Check sheet for the modelled part. Datum: model origin and axes. Units: mm. Coordinates: 2 decimals unless noted, no trailing zeros. Loops run counter-clockwise (first coordinate to the right, second up) from the corner with the lowest first, then second, coordinate; pieces in that order, holes last. Notation, with made-up numbers: (-1.75, -38.5) -> (22.25, -38.5) arc R10 ccw to (22.25, -26.5) -> close; hole circle Ø11 at (36.25, 12.25). An arc over 180 degrees is marked (long way). Use CSV: the item, a comma, the result in double quotes.
```python
from build123d import *

# Parameters (mm, degrees)
SKIZZE1_R                            = 20.35
SKIZZE1_R_2                          = 19
AUFSATZ_LINEAR_AUSTRAGEN1_DEPTH      = 170
SKIZZE2_R                            = 2.5
SCHNITT_LINEAR_AUSTRAGEN1_DEPTH      = 21.35
SCHNITT_LINEAR_AUSTRAGEN1_DEPTH_BACK = 21.35
SKIZZE3_R                            = 2.5
SCHNITT_LINEAR_AUSTRAGEN2_DEPTH      = 21.3500001
SCHNITT_LINEAR_AUSTRAGEN2_DEPTH_BACK = 21.3500001


with BuildPart() as part:
    # Skizze1 → Aufsatz-Linear austragen1 (new body)
    with BuildSketch(Plane(origin=(0, 0, 0), x_dir=(1, 0, 0), z_dir=(0, 1, 0))):
        Circle(SKIZZE1_R)
        Circle(SKIZZE1_R_2, mode=Mode.SUBTRACT)
    extrude(amount=AUFSATZ_LINEAR_AUSTRAGEN1_DEPTH)

    # Skizze2 → Schnitt-Linear austragen1 (cut, two sides)
    with BuildSketch(Plane.XY) as schnitt_linear_austragen1_sk:
        with Locations((0, 162.5)):
            Circle(SKIZZE2_R)
    extrude(amount=SCHNITT_LINEAR_AUSTRAGEN1_DEPTH, mode=Mode.SUBTRACT)
    extrude(schnitt_linear_austragen1_sk.sketch, amount=-SCHNITT_LINEAR_AUSTRAGEN1_DEPTH_BACK, mode=Mode.SUBTRACT)

    # Skizze3 → Schnitt-Linear austragen2 (cut, two sides)
    with BuildSketch(Plane(origin=(0, 0, 0), x_dir=(0, 0, -1), z_dir=(1, 0, 0))) as schnitt_linear_austragen2_sk:
        with Locations((0, 162.5)):
            Circle(SKIZZE3_R)
    extrude(amount=SCHNITT_LINEAR_AUSTRAGEN2_DEPTH, mode=Mode.SUBTRACT)
    extrude(schnitt_linear_austragen2_sk.sketch, amount=-SCHNITT_LINEAR_AUSTRAGEN2_DEPTH_BACK, mode=Mode.SUBTRACT)


solid = part.part
```
1) Cross-section at C-C on z = -9. Record the boundary of the cut face in (x, y).
Answer below:
outline,"(-18.25, 0) -> (-16.73, 0) -> (-16.73, 170) -> (-18.25, 170) -> close; (16.73, 0) -> (18.25, 0) -> (18.25, 170) -> (16.73, 170) -> close"
2) Draft check along Y on faces 1 (the flat face through (-17, 170, -9)), 2 (the flat face through (-17, 0, -9)), 3 (the cylindrical face through (20, 165, 0)). Enter one of: released by +Y, released by -Y, zero draft, split by the parting line, or undercut.
Answer below:
face 1,"released by +Y"
face 2,"released by -Y"
face 3,"undercut"
3) Cross-section at A-A on z = 0. Record the boundary of the cut face in (x, y), and give its area (4 significant figures).
Answer below:
outline,"(-20.35, 0) -> (-19, 0) -> (-19, 160) -> (-20.35, 160) -> close; (-20.35, 165) -> (-19, 165) -> (-19, 170) -> (-20.35, 170) -> close; (19, 0) -> (20.35, 0) -> (20.35, 160) -> (19, 160) -> close; (19, 165) -> (20.35, 165) -> (20.35, 170) -> (19, 170) -> close"
area,"445.5 mm²"
4) Cross-section at B-B on x = 0. Record the boundary of the cut face in (y, z), and give its area (4 significant figures).
Answer below:
outline,"(0, -20.35) -> (160, -20.35) -> (160, -19) -> (0, -19) -> close; (0, 19) -> (160, 19) -> (160, 20.35) -> (0, 20.35) -> close; (165, -20.35) -> (170, -20.35) -> (170, -19) -> (165, -19) -> close; (165, 19) -> (170, 19) -> (170, 20.35) -> (165, 20.35) -> close"
area,"445.5 mm²"
5) Go/stop test with flat-tipped pins: pin 1 Ø1.5 at (y, z) = (75, -13.5) entering from -X; pin 2 Ø2 at (y, z) = (109.5, 13.5) entering from +X; pin 3 Ø1.5 at (y, z) = (75.5, -6.5) entering from -X. Record where each tip stops, or that it passes through.
Answer below:
pin 1,"stops at x = -15.86"
pin 2,"stops at x = 16.06"
pin 3,"stops at x = -19.52"
6) Thickness scan on line 1 along Z through (x, y) = (0, 74); line 2 along Y through (x, z) = (-19.25, 0); line 3 along X through (y, z) = (129, 1). Record the ranges inside material, lowest first. Write a range as from..to.
Answer below:
line 1,"z = -20.35..-19, 19..20.35"
line 2,"y = 0..160, 165..170"
line 3,"x = -20.33..-18.97, 18.97..20.33"
7) Cross-section at D-D on x = 9. Record the boundary of the cut face in (y, z).
Answer below:
outline,"(0, -18.25) -> (170, -18.25) -> (170, -16.73) -> (0, -16.73) -> close; (0, 16.73) -> (170, 16.73) -> (170, 18.25) -> (0, 18.25) -> close"
